from build123d import *

# Parameters (mm, degrees)
BOSS_EXTRUDE1_DEPTH      = 35
BOSS_EXTRUDE1_DEPTH_BACK = 35
SKETCH2_R                = 10
CUT_EXTRUDE1_DEPTH       = 35
SKETCH3_R                = 7.5
CUT_EXTRUDE2_DEPTH       = 80.78895104
FILLET1_R                = 30
FILLET2_R                = 10


with BuildPart() as part:
    # Sketch1 → Boss-Extrude1 (new body, two sides)
    with BuildSketch(Plane(origin=(0, 0, 0), x_dir=(0, 0, -1), z_dir=(1, 0, 0))) as boss_extrude1_sk:
        Polygon((-42.056921018, 166.399972685), (-42.056921018, 60.21769331), (-28.717037647, 60.21769331), (-28.717037647, 200.21769331), (37.732030022, 200.21769331), (37.732030022, 210.21769331), (-42.056921018, 210.21769331), align=None)
    extrude(amount=BOSS_EXTRUDE1_DEPTH)
    extrude(boss_extrude1_sk.sketch, amount=-BOSS_EXTRUDE1_DEPTH_BACK)

    # Sketch2 → Cut-Extrude1 (cut)
    with BuildSketch(Plane(origin=(0, 210.21769331, 0), x_dir=(1, 0, 0), z_dir=(0, 1, 0))):
        with Locations((0, -2.5)):
            Circle(SKETCH2_R)
    extrude(amount=-CUT_EXTRUDE1_DEPTH, mode=Mode.SUBTRACT)

    # Sketch3 → Cut-Extrude2 (cut, through all)
    with BuildSketch(Plane.XY.offset(42.056921018)):
        with Locations((0, 78.21769331)):
            Circle(SKETCH3_R)
    extrude(amount=-CUT_EXTRUDE2_DEPTH, mode=Mode.SUBTRACT)

    # Fillet1
    fillet1_edges = [part.edges().sort_by_distance(p)[0] for p in [
        (-35, 60.21769331, 35.386979332),
        (35, 60.21769331, 35.386979332),
        (35, 205.21769331, -37.732030022),
        (-35, 205.21769331, -37.732030022),
    ]]
    fillet(fillet1_edges, radius=FILLET1_R)

    # Fillet2
    fillet2_edges = [part.edges().sort_by_distance(p)[0] for p in [
        (0, 210.21769331, 42.056921018),
        (0, 200.21769331, 28.717037647),
    ]]
    fillet(fillet2_edges, radius=FILLET2_R)


solid = part.part
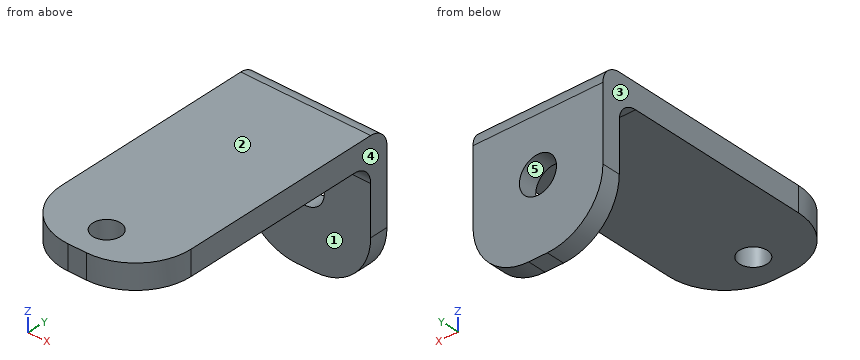
Work out the finished part from the listing and answer in its coordinate system (mm). Face numbers are marked on the shaded views. A direction names the side the tool comes from. Coordinates: 2 decimals unless noted, no trailing zeros. Write each loop counter-clockwise with the first axis right and the second up, starting at its lowest first coordinate (ties: lowest second). Pieces come first, ordered by that corner, then holes. Notation, with made-up numbers: M 64,53 L 86,53 A12 cw 86,61 Z; hole C -34.75,72 d11. An arc over 180 degrees is marked long. Use one line per item in the form item = value. Start each with the question number.
1. The part is cut by section B-B (z = 2.5). Give the vertices of the cut face in (x, y), plus the area to 3 significant figures.
2. Each of these flat-tipped pins is pushed along its axis until it touches: P1, Ø13.5, axis at x = 0, y = 78.22, coming from the -Z side; P2, Ø21, axis at x = -4.5, y = 141.5, coming from the -Z side. Where does it stop, or does it pass through?
3. The part is cut by section C-C (x = -22). Give the vertices of the cut face in (y, z).
4. Straight lines are drawn through the part: probe 1 along Y at (x, z) = (0, 31.75); probe 2 along Z at (x, y) = (-2, 177.5); probe 3 along Y at (x, z) = (-11, 1). For each, find the intervals that lie inside material, in ascending order. Write a range as from..to.
5. The part is cut by section A-A (x = 0). Give the vertices of the cut face in (y, z), plus the area to 3 significant figures.
6. The part is cut by section D-D (y = 112). Give the vertices of the cut face in (x, z).
7. A tool of negligible diameter and unlimited length cuts with its end or side. For the marked faces 1 and 2, from which of +Z, -Z, +X, -X, +Y, -Y can it reach the whole face along a straight path? Write none if from no direction.
8. The mould has two halves that part along X. Classify the marked faces 3, 4 and 5: released by +X, released by -X, zero draft, split by the parting line, or undercut.
Evaluation:
q1.outline = M -35,200.22 L -10,200.22 L -10,210.22 L -35,210.22 Z; M 10,200.22 L 35,200.22 L 35,210.22 L 10,210.22 Z
q1.area = 500 mm^2
q2.P1 = through
q2.P2 = 28.72
q3.outline = M 65.5,28.72 L 190.22,28.72 A10 cw 200.22,18.72 L 200.22,-32.45 L 210.22,-32.45 L 210.22,32.06 A10 ccw 200.22,42.06 L 65.5,42.06 Z
q4.probe_1 = 60.22..70.72, 85.72..210.22
q4.probe_2 = 28.72..42.06
q4.probe_3 = 200.22..210.22
q5.outline = M 60.22,28.72 L 70.72,28.72 L 70.72,42.06 L 60.22,42.06 Z; M 85.72,28.72 L 190.22,28.72 A10 cw 200.22,18.72 L 200.22,12.5 L 210.22,12.5 L 210.22,32.06 A10 ccw 200.22,42.06 L 85.72,42.06 Z; M 200.22,-37.73 L 210.22,-37.73 L 210.22,-7.5 L 200.22,-7.5 Z
q5.area = 2,270 mm^2
q6.outline = M -35,28.72 L 35,28.72 L 35,42.06 L -35,42.06 Z
q7.face_1 = -Z, +X, -X, -Y
q7.face_2 = +Z, +X, -X, +Y, -Y
q8.face_3 = released by -X
q8.face_4 = released by +X
q8.face_5 = undercut
